Model file for the job. Use its own axes, mm. Face numbers are marked on the shaded views. Give positions to 0.01 mm unless a question says otherwise; leave off trailing zeros. Loops run counter-clockwise (first coordinate to the right, second up) from the corner with the lowest first, then second, coordinate; pieces in that order, holes last. Notation, with made-up numbers: M 23.5,-16 L 72.5,-16 A17 ccw 72.5,1 Z; hole C 57.25,-12.5 d3. An arc over 180 degrees is marked long. Answer in a Markdown table with one row per item.
```python
from build123d import *

# Parameters (mm, degrees)
BOSS_EXTRUDE1_DEPTH = 2
SKETCH2_R           = 4.3
SKETCH2_R_2         = 2.9
BOSS_EXTRUDE2_DEPTH = 3
SKETCH3_R           = 1.5
CUT_EXTRUDE1_DEPTH  = 3


with BuildPart() as part:
    # Sketch1 → Boss-Extrude1 (new body)
    with BuildSketch(Plane.XY):
        with BuildLine():
            Line((-2.5, 18.85), (-4.222289698, 0.813799547))
            ThreePointArc((-4.222289698, 0.813799547), (-4.3, 0), (-4.222289698, -0.813799547))
            Line((-4.222289698, -0.813799547), (-2.5, -18.85))
            ThreePointArc((-2.5, -18.85), (0, -21.35), (2.5, -18.85))
            Line((2.5, -18.85), (4.222289698, -0.813799547))
            ThreePointArc((4.222289698, -0.813799547), (4.3, 0), (4.222289698, 0.813799547))
            Line((4.222289698, 0.813799547), (2.5, 18.85))
            ThreePointArc((2.5, 18.85), (0, 21.35), (-2.5, 18.85))
        make_face()
    extrude(amount=BOSS_EXTRUDE1_DEPTH)

    # Sketch2 → Boss-Extrude2 (add)
    with BuildSketch(Plane.XY.offset(2)):
        Circle(SKETCH2_R)
        Circle(SKETCH2_R_2, mode=Mode.SUBTRACT)
    extrude(amount=BOSS_EXTRUDE2_DEPTH)

    # Sketch3 → Cut-Extrude1 (cut, through all)
    with BuildSketch(Plane.XY.offset(2)):
        Circle(SKETCH3_R)
    extrude(amount=-CUT_EXTRUDE1_DEPTH, mode=Mode.SUBTRACT)


solid = part.part
```
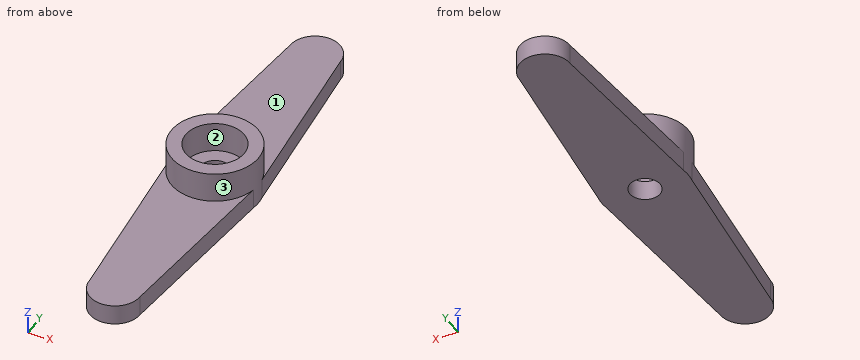
Q1. Saw through at D-D (y = 6.5). Give the cut face in (x, z).
Reported:
| item | result |
|---|---|
| outline | M -3.68,0 L 3.68,0 L 3.68,2 L -3.68,2 Z |
Q2. Saw through at A-A (x = 0). Give the cut face in (y, z), and give its area (3 significant figures).
Reported:
| item | result |
|---|---|
| outline | M -21.35,0 L -1.5,0 L -1.5,2 L -2.9,2 L -2.9,5 L -4.3,5 L -4.3,2 L -21.35,2 Z; M 1.5,0 L 21.35,0 L 21.35,2 L 4.3,2 L 4.3,5 L 2.9,5 L 2.9,2 L 1.5,2 Z |
| area | 87.8 mm² |
Q3. Probe probe 1 along X at (y, z) = (-19, 1.1); probe 2 along Y at (x, z) = (0, 0.7); probe 3 along Y at (x, z) = (0.25, 2.7). List the from-to ranges inside material, lowest first.
Reported:
| item | result |
|---|---|
| probe 1 | -2.5 to 2.5 |
| probe 2 | -21.35 to -1.5, 1.5 to 21.35 |
| probe 3 | -4.29 to -2.89, 2.89 to 4.29 |
Q4. Drop a flat-ended pin along its axis: pin 1 (2 mm diameter, centred on x = -3, y = -13, fed in from +Z). Give the stop position or say it passes through.
Reported:
| item | result |
|---|---|
| pin 1 | z = 2 |
Q5. Mould opens along Y. For the marked faces 1, 2 and 3 say: released by +Y, released by -Y, zero draft, split by the parting line, or undercut.
Reported:
| item | result |
|---|---|
| face 1 | zero draft |
| face 2 | undercut |
| face 3 | split by the parting line |
Q6. Saw through at C-C (y = -9.5). Give the cut face in (x, z), and give its area (3 significant figures).
Reported:
| item | result |
|---|---|
| outline | M -3.39,0 L 3.39,0 L 3.39,2 L -3.39,2 Z |
| area | 13.6 mm² |
Q7. Saw through at B-B (z = 3.1). Give the cut face in (x, y), and give its area (3 significant figures).
Reported:
| item | result |
|---|---|
| outline | C 0,0 d8.6; hole C 0,0 d5.8 |
| area | 31.7 mm² |
